Autodesk Inventor part; units mm, degrees
ref_plane "bracket_to_dummy_XY" through (0, 0, 0) normal (0, 1, 0) x (1, 0, 0)
ref_plane "bracket_to_dummy_YZ" through (0, 0, 0) normal (1, 0, 0) x (0, 0, -1)
ref_plane "bracket_to_dummy_ZX" through (0, 0, 0) normal (0, 0, -1) x (0, 1, 0)
sketch "Sketch_8" plane through (0, 0, 0) normal (1, 0, 0) x (0, 1, 0)
  line L0 (0, 70) -> (0, 0)
  line L1 (0, 0) -> (49.4975, -49.4975)
  line L2 (49.4975, -49.4975) -> (55.8614, -43.1335)
  line L3 (55.8614, -43.1335) -> (41.7193, -28.9914)
  line L4 (41.7193, -28.9914) -> (9, 49.9914)
  line L5 (9, 49.9914) -> (9, 70)
  line L6 (9, 70) -> (0, 70)
  arc A0 (23.0035, 5.74) -> (21.0437, 6.5518) centre (21.6177, 5.166) ccw
  line L7 (21.0437, 6.5518) -> (17.935, 5.2641)
  arc A1 (17.935, 5.2641) -> (17.0297, 4.1265) centre (18.509, 3.8783) ccw
  arc A2 (10.9882, -0.0281) -> (17.0297, 4.1265) centre (12, 4.9706) ccw
  arc A3 (10.9882, -0.0281) -> (9.63, -2.5589) centre (10.6906, -1.4983) ccw
  line L8 (9.63, -2.5589) -> (32.996, -25.9249)
  arc A4 (32.996, -25.9249) -> (35.4424, -24.2902) centre (34.0566, -24.8642) ccw
  line L9 (35.4424, -24.2902) -> (23.0035, 5.74)
  circle A5 centre (12, 4.9706) radius 2.1
  arc A6 (7.8859, 42.2372) -> (5.0029, 41.7559) centre (6.5, 41.6633) ccw
  line L10 (5.0029, 41.7559) -> (5, 8.619)
  arc A7 (5, 8.619) -> (7.7564, 7.7993) centre (6.5, 8.6189) ccw
  arc A8 (14.9597, 9.1239) -> (7.7564, 7.7993) centre (12, 4.9705) ccw
  arc A9 (14.9597, 9.1239) -> (16.4042, 8.9596) centre (15.8302, 10.3455) ccw
  line L11 (16.4042, 8.9596) -> (19.5129, 10.2473)
  arc A10 (19.5129, 10.2473) -> (20.3596, 12.1145) centre (18.9389, 11.6331) ccw
  line L12 (20.3596, 12.1145) -> (7.8859, 42.2372)
extrude "Extrusion1" add sketch "Sketch_8" along normal mid plane 20
sketch "Sketch_3" plane through (0, 0, 0) normal (0, 1, 0) x (-1, 0, 0)
  circle A0 centre (0, 60) radius 3.5
extrude "Extrusion2" cut sketch "Sketch_3" along normal blind 9
sketch "Sketch_9" plane through (0, 0, 0) normal (1, 0, 0) x (0, 1, 0)
  line L0 (42.4264, -42.4264) -> (48.7904, -36.0624)
  line L1 (48.7904, -36.0624) -> (51.2652, -38.5373)
  line L2 (51.2652, -38.5373) -> (44.9013, -44.9013)
  line L3 (44.9013, -44.9013) -> (42.4264, -42.4264)
  line L4 (42.4264, -42.4264) -> (48.7904, -36.0624)
revolve "Revolution1" cut sketch "Sketch_9" angle 360 about axis through (0, 42.4264, -42.4264) along (0, -0.7071, -0.7071)
ref_plane "bracket_to_dummy_XY" through (0, 0, 0) normal (0, 1, 0) x (1, 0, 0)
ref_plane "bracket_to_dummy_YZ" through (0, 0, 0) normal (1, 0, 0) x (0, 0, -1)
ref_plane "bracket_to_dummy_ZX" through (0, 0, 0) normal (0, 0, -1) x (0, 1, 0)
ref_plane "1_to_bolt_XY" through (0, 9, 60) normal (0, 1, 0) x (1, 0, 0)
ref_plane "1_to_bolt_YZ" through (0, 9, 60) normal (1, 0, 0) x (0, 0, -1)
ref_plane "1_to_bolt_ZX" through (0, 9, 60) normal (0, 0, -1) x (0, 1, 0)
ref_plane "6_to_bolt_XY" through (0, 48.7904, -36.0624) normal (0, 0.7071, 0.7071) x (0, 0.7071, -0.7071)
ref_plane "6_to_bolt_YZ" through (0, 48.7904, -36.0624) normal (0, 0.7071, -0.7071) x (-1, 0, 0)
ref_plane "6_to_bolt_ZX" through (0, 48.7904, -36.0624) normal (-1, 0, 0) x (0, 0.7071, 0.7071)
ref_plane "7_to_bolt_XY" through (30, 48.7904, -36.0624) normal (0, 0.7071, 0.7071) x (0, 0.7071, -0.7071)
ref_plane "7_to_bolt_YZ" through (30, 48.7904, -36.0624) normal (0, 0.7071, -0.7071) x (-1, 0, 0)
ref_plane "7_to_bolt_ZX" through (30, 48.7904, -36.0624) normal (-1, 0, 0) x (0, 0.7071, 0.7071)
ref_plane "8_to_bolt_XY" through (0, 9, 60) normal (0, 1, 0) x (0, 0, -1)
ref_plane "8_to_bolt_YZ" through (0, 9, 60) normal (0, 0, -1) x (-1, 0, 0)
ref_plane "8_to_bolt_ZX" through (0, 9, 60) normal (-1, 0, 0) x (0, 1, 0)
ref_plane "9_to_bolt_XY" through (30, 9, 60) normal (0, 1, 0) x (0, 0, -1)
ref_plane "9_to_bolt_YZ" through (30, 9, 60) normal (0, 0, -1) x (-1, 0, 0)
ref_plane "9_to_bolt_ZX" through (30, 9, 60) normal (-1, 0, 0) x (0, 1, 0)
properties part number "HBL135TS6hbl45ts6"
Could you check a few things on this model? Use its own coordinates, in mm. A direction names the side the tool comes from. Round coordinates to 2 decimals unless told otherwise and drop trailing zeros. Loops run counter-clockwise (first coordinate to the right, second up) from the corner with the lowest first, then second, coordinate; pieces in that order, holes last. Notation, with made-up numbers: (76, -17) - (128, -17) arc R13 ccw to (128, -6) - close; hole circle Ø1 at (-32.75, 33.5). An arc over 180 degrees is marked (long way). Write item = value, one per line.
1) Imagine slicing it at C-C (y = 31). Please give me the cut outline in (x, z).
Computed:
outline = (-10, -31) - (10, -31) - (10, -23.93) - (-10, -23.93) - close; (-10, -13.57) - (10, -13.57) - (10, -3.12) - (-10, -3.12) - close
2) Imagine slicing it at B-B (z = 60). Please give me the cut outline in (x, y), and give its area (3 significant figures).
Computed:
outline = (-10, 0) - (-3.5, 0) - (-3.5, 9) - (-10, 9) - close; (3.5, 0) - (10, 0) - (10, 9) - (3.5, 9) - close
area = 117 mm2
3) I'm going to push flat-ended pins straight in: P1, Ø6, axis at x = -2.5, z = -23.5, coming from the -Y side; P2, Ø1.5, axis at x = 2, y = 29.5, coming from the +Z side; P3, Ø12, axis at x = -2.5, y = 26.5, coming from the -Z side. Where does each tip first touch, or does it pass through?
Computed:
P1 = 20.5
P2 = 2.32
P3 = -32.5
4) On a 3-axis mill with a long thin cutter (end or side, diameter ignored), from which of +Z, -Z, +X, -X, +Y, -Y can I reach the whole of each face in a straight line? I mean faces 1 (the flat face through (0, 0, 35)), 2 (the flat face through (-0.14, 14.21, 26.96)), 3 (the flat face through (-5, 9, 60)). Say none if no direction works.
Computed:
face_1 = +Z, -Z, +X, -X, -Y
face_2 = +X, -X
face_3 = +Z, +X, -X, +Y
5) If we mould it in two halves opening along Z, with no side actions, what happens to faces 4 (the flat face through (-0.14, 52.635, -46.36)), 5 (the flat face through (0, 5, 70)), 6 (the cylindrical face through (-0.1, 9.9, 4.9))? For each: pulls with the +Z half, pulls with the -Z half, needs draft (parallel to the pull), parting line crosses it, or undercut.
Computed:
face_4 = pulls with the -Z half
face_5 = pulls with the +Z half
face_6 = undercut
6) Imagine slicing it at D-D (x = 5.5). Please give me the cut outline in (y, z) (1 decimal), and give its area (3 significant figures).
Computed:
outline = (0, 0) - (49.5, -49.5) - (55.9, -43.1) - (41.7, -29) - (9, 50) - (9, 70) - (0, 70) - close; hole (5, 8.6) arc R1.5 ccw to (7.8, 7.8) arc R5.1 cw to (15, 9.1) arc R1.5 ccw to (16.4, 9) - (19.5, 10.2) arc R1.5 ccw to (20.4, 12.1) - (7.9, 42.2) arc R1.5 ccw to (5, 41.8) - close; hole (9.6, -2.6) - (33, -25.9) arc R1.5 ccw to (35.4, -24.3) - (23, 5.7) arc R1.5 ccw to (21, 6.6) - (17.9, 5.3) arc R1.5 ccw to (17, 4.1) arc R5.1 cw to (11, 0) arc R1.5 ccw to start; hole circle Ø4.2 at (12, 5)
area = 1,330 mm2
7) Imagine slicing it at A-A (x = 0). Give the number of separate pieces and of enclosed holes in the cut face, and give its area (3 significant figures).
Computed:
separate_pieces = 3
enclosed_holes = 3
area = 1,200 mm2
8) I need wall thicknesses on line 1 along Z through (x, y) = (0, 3.5); line 2 along Z through (x, y) = (1.25, 20); line 3 along Y through (x, z) = (-2, 6). Which ranges of each line are inside material? Lowest first, please. Write a range as from..to.
Computed:
line_1 = -3.5..56.5, 63.5..70
line_2 = -20..-12.93, 6.12..10.57, 12.98..23.44
line_3 = 0..10.17, 13.83..19.71, 22.86..27.22
